```python
from build123d import *

# Parameters (mm, degrees)
SKETCH_1_W                = 680
SKETCH_1_H                = 480
EXTRUDE_1_DEPTH           = 20
FILLET_1_R                = 9
CHAMFER_3_SIZE            = 2
HOLE_WIZARD_M30_1_D       = 26.5
HOLE_WIZARD_M30_1_DEPTH   = 70.5
HOLE_WIZARD_M30_1_TIP     = 7.961403202
HOLE_WIZARD_M8_1_D        = 6.8
HOLE_WIZARD_2_D           = 6.6
HOLE_WIZARD_2_DEPTH       = 19.75
HOLE_WIZARD_2_CBORE_D     = 11
HOLE_WIZARD_2_CBORE_DEPTH = 6.8
HOLE_WIZARD_2_TIP         = 1.982840043
HOLE_WIZARD_3_D           = 13.5
HOLE_WIZARD_3_DEPTH       = 19.75
HOLE_WIZARD_3_CBORE_D     = 20
HOLE_WIZARD_3_CBORE_DEPTH = 13
HOLE_WIZARD_3_TIP         = 4.055809178
HOLE_WIZARD_M8_2_D        = 6.8


with BuildPart() as part:
    # 草图1 → 凸台-拉伸1 (new body)
    with BuildSketch(Plane.XY):
        Rectangle(SKETCH_1_W, SKETCH_1_H)
    extrude(amount=EXTRUDE_1_DEPTH)

    # 圆角1
    fillet_1_edges = [part.edges().sort_by_distance(p)[0] for p in [
        (340, -240, 10),
        (-340, -240, 10),
        (-340, 240, 10),
        (340, 240, 10),
    ]]
    fillet(fillet_1_edges, radius=FILLET_1_R)

    # 倒角3
    chamfer_3_edges = [part.edges().sort_by_distance(p)[0] for p in [
        (-340, 0, 0),
        (-340, 0, 20),
        (340, 0, 0),
        (0, -240, 0),
        (0, 240, 0),
        (-337.363961031, -237.363961031, 0),
        (337.363961031, -237.363961031, 0),
        (337.363961031, 237.363961031, 0),
        (-337.363961031, 237.363961031, 0),
        (0, 240, 20),
        (340, 0, 20),
        (0, -240, 20),
        (-337.363961031, -237.363961031, 20),
        (337.363961031, -237.363961031, 20),
        (337.363961031, 237.363961031, 20),
        (-337.363961031, 237.363961031, 20),
    ]]
    chamfer(chamfer_3_edges, length=CHAMFER_3_SIZE)

    # M30 螺纹孔1
    with Locations(Plane(origin=(0, 0, 0), x_dir=(-1, 0, 0), z_dir=(0, 0, -1))):
        with Locations((0, 210), (-310, 0), (0, -210), (310, 0)):
            Hole(HOLE_WIZARD_M30_1_D / 2, depth=HOLE_WIZARD_M30_1_DEPTH)
            with Locations((0, 0, -(HOLE_WIZARD_M30_1_DEPTH + HOLE_WIZARD_M30_1_TIP / 2))):  # 118° drill point
                Cone(0, HOLE_WIZARD_M30_1_D / 2, HOLE_WIZARD_M30_1_TIP, mode=Mode.SUBTRACT)

    # M8 螺纹孔1 (through all)
    with Locations(Plane(origin=(0, 0, 0), x_dir=(-1, 0, 0), z_dir=(0, 0, -1))):
        with Locations((330.25, -231.25), (285.75, -231.25), (285.75, -156.75), (330.25, -156.75), (-285.75, -231.25), (-330.25, -231.25), (-330.25, -156.75), (-285.75, -156.75), (330.25, 156.75), (285.75, 156.75), (285.75, 231.25), (330.25, 231.25), (-285.75, 156.75), (-330.25, 156.75), (-330.25, 231.25), (-285.75, 231.25)):
            Hole(HOLE_WIZARD_M8_1_D / 2)

    # 打孔尺寸(%根据)内六角圆柱头螺钉的类型2
    with Locations(Plane(origin=(0, 0, 0), x_dir=(-1, 0, 0), z_dir=(0, 0, -1))):
        with Locations((225, -210), (75, -210), (-75, -210), (-225, -210), (225, 210), (75, 210), (-75, 210), (-225, 210), (310, -175), (310, 175), (-310, -175), (-310, 175), (-310, -75), (-310, 75), (310, -75), (310, 75)):
            CounterBoreHole(HOLE_WIZARD_2_D / 2, HOLE_WIZARD_2_CBORE_D / 2, HOLE_WIZARD_2_CBORE_DEPTH, depth=HOLE_WIZARD_2_DEPTH)
            with Locations((0, 0, -(HOLE_WIZARD_2_DEPTH + HOLE_WIZARD_2_TIP / 2))):  # 118° drill point
                Cone(0, HOLE_WIZARD_2_D / 2, HOLE_WIZARD_2_TIP, mode=Mode.SUBTRACT)

    # 打孔尺寸(%根据)内六角圆柱头螺钉的类型3
    with Locations(Plane(origin=(0, 0, 0), x_dir=(-1, 0, 0), z_dir=(0, 0, -1))):
        with Locations((78.500000006, -135.000000012), (-78.499999994, -135.000000012), (-78.499999994, 134.999999988), (78.500000006, 134.999999988)):
            CounterBoreHole(HOLE_WIZARD_3_D / 2, HOLE_WIZARD_3_CBORE_D / 2, HOLE_WIZARD_3_CBORE_DEPTH, depth=HOLE_WIZARD_3_DEPTH)
            with Locations((0, 0, -(HOLE_WIZARD_3_DEPTH + HOLE_WIZARD_3_TIP / 2))):  # 118° drill point
                Cone(0, HOLE_WIZARD_3_D / 2, HOLE_WIZARD_3_TIP, mode=Mode.SUBTRACT)

    # M8 螺纹孔2 (through all)
    with Locations(Plane.XY.offset(20)):
        with Locations((-173.5, 135.000000012), (-78.5, 40.000000013), (173.5, 135.000000012), (78.5, 40.000000013), (78.499999997, -39.999999988), (-78.500000003, -39.999999988), (-173.5, -134.999999988), (173.5, -134.999999988)):
            Hole(HOLE_WIZARD_M8_2_D / 2)


solid = part.part
```
Here's how the part is built. I have some questions about the finished solid (model axes, mm). A direction names the side the tool comes from. Coordinates: 2 decimals unless noted, no trailing zeros. Order: outer loops, then holes, each group sorted by start corner. A loop starts at its lowest first (then second) coordinate and runs counter-clockwise, first axis right, second up. Notation, with made-up numbers: (-4.75, -8.5) -> (14.25, -8.5) arc R22 ccw to (14.25, -0.5) -> close; hole circle Ø6 at (46, 26). An arc over 180 degrees is marked (long way). Return JSON: item names as keys, results as strings.
1) If we section it at A-A on x = 0: List the corners of the cut face in (y, z) for me, plus the area to 3 significant figures.
Conclusion:
{"outline": "(-240, 2) -> (-238, 0) -> (-223.25, 0) -> (-223.25, 20) -> (-238, 20) -> (-240, 18) -> close; (-196.75, 0) -> (196.75, 0) -> (196.75, 20) -> (-196.75, 20) -> close; (223.25, 0) -> (238, 0) -> (240, 2) -> (240, 18) -> (238, 20) -> (223.25, 20) -> close", "area": "8,530 mm²"}
2) Thinking about a two-plate mould opening in Y: for faces 1 (the cylindrical face through (-75.39, 129.01, 16.42)), 2 (the flat face through (-5, 3, 0)), 3 (the cylindrical face through (-75.39, -140.99, 16.42)), which applies, +Y half, -Y half, draft (parallel to the pull), parting line (faces both ways), or undercut?
Conclusion:
{"face 1": "undercut", "face 2": "draft", "face 3": "undercut"}
3) On a 3-axis mill with a long thin cutter (end or side, diameter ignored), from which of +Z, -Z, +X, -X, +Y, -Y can I reach the whole of each face in a straight line? I mean faces 4 (the flat face through (-340, -3, 10)), 5 (the flat face through (-81, -142, 13)). Say none if no direction works.
Conclusion:
{"face 4": "+Z, -Z, -X, +Y, -Y", "face 5": "-Z"}
4) I'm going to push flat-ended pins straight in: P1, Ø3.5, axis at x = 312.5, y = -173, coming from the -Z side; P2, Ø6.5, axis at x = -310, y = 75, coming from the -Z side. Where does each tip first touch, or does it pass through?
Conclusion:
{"P1": "stops at z = 6.8", "P2": "stops at z = 19.78"}
5) If I drill on probe 1 along X at (y, z) = (75, 10.75); probe 2 along Y at (x, z) = (310, 4.75); probe 3 along Y at (x, z) = (-78.5, 7.75), over which ranges is the centre line in solid material (lowest first)?
Conclusion:
{"probe 1": "x = -340 to -313.3, -306.7 to 306.7, 313.3 to 340", "probe 2": "y = -240 to -180.5, -169.5 to -80.5, -69.5 to -13.25, 13.25 to 69.5, 80.5 to 169.5, 180.5 to 240", "probe 3": "y = -240 to -145, -125 to -43.4, -36.6 to 36.6, 43.4 to 125, 145 to 240"}
